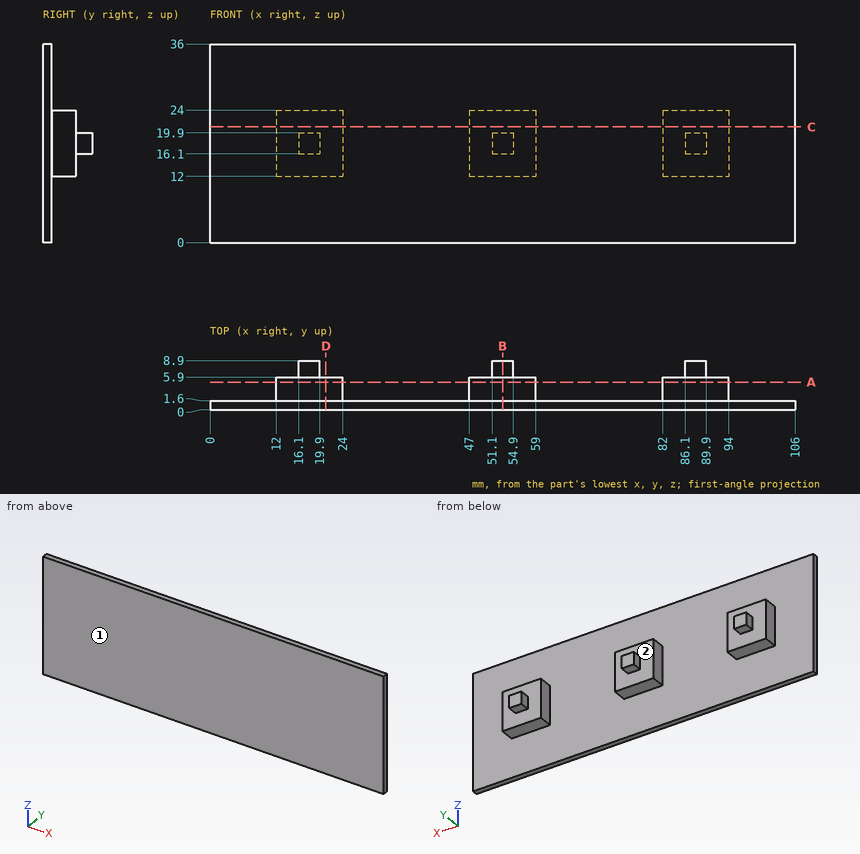
Source: three-view drawing plus pictorial views. Frame: mm from the lowest corner of the part. Give positions to 0.01 mm unless a question says otherwise; leave off trailing zeros. Loops run counter-clockwise (first coordinate to the right, second up) from the corner with the lowest first, then second, coordinate; pieces in that order, holes last. Notation, with made-up numbers: (82, -35.5) -> (136, -35.5) arc R10 ccw to (136, -17.5) -> close; hole circle Ø5 at (58.25, 68.25). An arc over 180 degrees is marked (long way). Use a Markdown table: item, result. Add a question column.
(1) Section query C-C (z = 21). Output: boundary loops of the cut face in (x, y).
(2) Pull-direction query (X, two-part tool) for the marked faces 1 and 2; classes: +X half, -X half, draft (parallel to the pull), parting line (faces both ways), or undercut.
(3) Section query D-D (x = 21). Output: boundary loops of the cut face in (y, z).
(4) First-contact query: pin 1 Ø3 at (y, z) = (3.5, 28.5) entering from -X; pin 2 Ø4 at (x, z) = (49.5, 4) entering from +Y; pin 3 Ø3.5 at (y, z) = (7.5, 18) entering from +X; pin 4 Ø4.5 at (x, y) = (55.5, 4.5) entering from +Z. Flat tips, straight axial feed; report the tip coordinate or a pass-through.
(5) Section query A-A (y = 5). Output: boundary loops of the cut face in (x, z).
(6) Section query B-B (x = 53). Output: boundary loops of the cut face in (y, z), then the cut area to 3 significant figures.
(7) Ray query, line 1 (X direction, y = 4, z = 22); line 2 (Y direction, x = 62, z = 13); line 3 (Z direction, x = 54, y = 7). Return the intervals inside material, ascending.
Checked values:
| question | item | result |
|---|---|---|
| 1 | outline | (0, 0) -> (106, 0) -> (106, 1.6) -> (94, 1.6) -> (94, 5.9) -> (82, 5.9) -> (82, 1.6) -> (59, 1.6) -> (59, 5.9) -> (47, 5.9) -> (47, 1.6) -> (24, 1.6) -> (24, 5.9) -> (12, 5.9) -> (12, 1.6) -> (0, 1.6) -> close |
| 2 | face 1 | draft |
| 2 | face 2 | undercut |
| 3 | outline | (0, 0) -> (1.6, 0) -> (1.6, 12) -> (5.9, 12) -> (5.9, 24) -> (1.6, 24) -> (1.6, 36) -> (0, 36) -> close |
| 4 | pin 1 | through |
| 4 | pin 2 | y = 1.6 |
| 4 | pin 3 | x = 94 |
| 4 | pin 4 | z = 24 |
| 5 | outline | (12, 12) -> (24, 12) -> (24, 24) -> (12, 24) -> close; (47, 12) -> (59, 12) -> (59, 24) -> (47, 24) -> close; (82, 12) -> (94, 12) -> (94, 24) -> (82, 24) -> close |
| 6 | outline | (0, 0) -> (1.6, 0) -> (1.6, 12) -> (5.9, 12) -> (5.9, 16.1) -> (8.9, 16.1) -> (8.9, 19.9) -> (5.9, 19.9) -> (5.9, 24) -> (1.6, 24) -> (1.6, 36) -> (0, 36) -> close |
| 6 | area | 121 mm^2 |
| 7 | line 1 | 12 to 24, 47 to 59, 82 to 94 |
| 7 | line 2 | 0 to 1.6 |
| 7 | line 3 | 16.1 to 19.9 |
